The listing builds one solid part. Answer for the finished solid, in the listing's coordinates (mm). Round coordinates to 2 decimals unless told otherwise and drop trailing zeros. Order: outer loops, then holes, each group sorted by start corner. A loop starts at its lowest first (then second) coordinate and runs counter-clockwise, first axis right, second up. Notation, with made-up numbers: (2, 68.25) - (32, 68.25) arc R28 ccw to (32, 91.25) - close; hole circle Ø7 at (13, 32). An arc over 180 degrees is marked (long way). Write item = value, one per line.
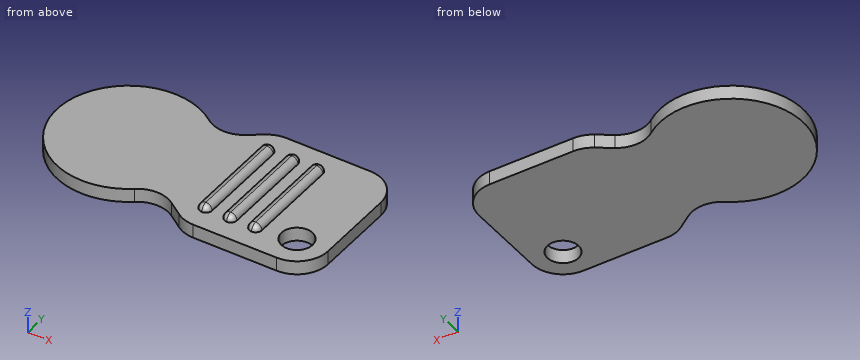
from build123d import *

# Parameters (mm, degrees)
F0_R     = 11.5
F1_DEPTH = 2.2
F3_DEPTH = 2.2
F4_R     = 2.5
F5_DEPTH = 2.201
F6_R     = 5
F7_W     = 2
F7_H     = 17
F8_DEPTH = 1
F9_R     = 0.99999


# Not quite as in the source:
# - a fillet or chamfer is up to 0.001 mm smaller than in the source, because OpenCascade refuses the exact size


with BuildPart() as f1:
    # F0 (on Top) → F1 (new body)
    with BuildSketch(Plane.XY):
        Circle(F0_R)
    extrude(amount=F1_DEPTH)

    # F2 (on Top) → F3 (join)
    with BuildSketch(Plane.XY):
        Polygon((16.363068172, 11.5), (0, 0), (16.363068172, -11.5), (36.363068172, -11.5), (36.363068172, 11.5), align=None)
    extrude(amount=F3_DEPTH)

    # F4 (on face) → F5 (cut, through all)
    with BuildSketch(Plane(origin=(0, 0, 0), x_dir=(1, 0, 0), z_dir=(0, 0, -1))):
        with Locations((31.363068172, 6.5)):
            Circle(F4_R)
    extrude(amount=-F5_DEPTH, mode=Mode.SUBTRACT)

    # F6
    f6_edges = [f1.edges().sort_by_distance(p)[0] for p in [
        (36.363068, -11.5, 1.1),
        (36.363068, 11.5, 1.1),
        (16.363068, -11.5, 1.1),
        (9.408764, -6.6125, 1.1),
        (9.408764, 6.6125, 1.1),
        (16.363068, 11.5, 1.1),
    ]]
    fillet(f6_edges, radius=F6_R)

    # F7 (on face) → F8 (join)
    with BuildSketch(Plane.XY.offset(2.2)):
        with Locations((17.363068172, 0)):
            Rectangle(F7_W, F7_H)
        with Locations((21.363068172, 0)):
            Rectangle(F7_W, F7_H)
        with Locations((25.363068172, 0)):
            Rectangle(F7_W, F7_H)
    extrude(amount=F8_DEPTH)

    # F9 (radius 1 in the source; OpenCascade refuses exactly that, so slightly less here)
    f9_edges = [f1.edges().sort_by_distance(p)[0] for p in [
        (16.363068, -8.5, 2.7),
        (18.363068, -8.5, 2.7),
        (20.363068, -8.5, 2.7),
        (22.363068, -8.5, 2.7),
        (24.363068, -8.5, 2.7),
        (26.363068, -8.5, 2.7),
        (26.363068, 8.5, 2.7),
        (16.363068, 8.5, 2.7),
        (24.363068, 8.5, 2.7),
        (22.363068, 8.5, 2.7),
        (18.363068, 8.5, 2.7),
        (20.363068, 8.5, 2.7),
        (20.363068, 0, 3.2),
        (22.363068, 0, 3.2),
        (21.363068, 8.5, 3.2),
        (21.363068, -8.5, 3.2),
        (18.363068, 0, 3.2),
        (16.363068, 0, 3.2),
        (17.363068, 8.5, 3.2),
        (17.363068, -8.5, 3.2),
        (26.363068, 0, 3.2),
        (24.363068, 0, 3.2),
        (25.363068, 8.5, 3.2),
        (25.363068, -8.5, 3.2),
    ]]
    fillet(f9_edges, radius=F9_R)


solid = f1.part
Q1. Section B-B on x = 0 is taken. Determine the outline of the cut face in (y, z).
Model answer:
outline = (-11.5, 0) - (11.5, 0) - (11.5, 2.2) - (-11.5, 2.2) - close
Q2. A flat-ended cylindrical pin translates along its axis: P1, Ø4, axis at x = 31.36, y = -6.5, coming from the -Z side. Find the tip coordinate at first contact, or state that the pin passes through.
Model answer:
P1 = through
Q3. Find the intervals of material crossed by line 1 (X direction, y = 7.5, z = 2.7); line 2 (Z direction, x = -8.5, y = -2.75); line 3 (X direction, y = -9.5, z = 1), in increasing order. Write a range as from..to.
Model answer:
line_1 = 16.5..18.23, 20.5..22.23, 24.5..26.23
line_2 = 0..2.2
line_3 = -6.48..6.48, 13.52..35.36
